from build123d import *

# Parameters (mm, degrees)
SKETCH2_W           = 25.4
SKETCH2_H           = 25.4
BOSS_EXTRUDE1_DEPTH = 25.4
SHELL1_T            = -4.7625
FILLET1_R           = 4.7625
SKETCH3_R           = 3.81
CUT_EXTRUDE1_DEPTH  = 25.4


with BuildPart() as part:
    # Sketch2 → Boss-Extrude1 (new body)
    with BuildSketch(Plane.XY):
        with Locations((12.7, 12.7)):
            Rectangle(SKETCH2_W, SKETCH2_H)
    extrude(amount=BOSS_EXTRUDE1_DEPTH)

    # Shell1
    shell1_openings = [part.faces().sort_by_distance(p)[0] for p in [
        (12.7, 12.7, 25.4),
        (12.7, 12.7, 0),
        (12.7, 25.4, 12.7),
        (25.4, 12.7, 12.7),
    ]]
    offset(amount=SHELL1_T, openings=shell1_openings, kind=Kind.INTERSECTION)

    # Fillet1
    fillet1_edges = [part.edges().sort_by_distance(p)[0] for p in [
        (25.4, 4.7625, 12.7),
        (4.7625, 25.4, 12.7),
    ]]
    fillet(fillet1_edges, radius=FILLET1_R - 0.0001)  # a hair under: the kernel refuses the full size

    # Sketch3 → Cut-Extrude1 (cut)
    with BuildSketch(Plane.ZY):
        with Locations((12.7, 12.7)):
            Circle(SKETCH3_R)
    cut_extrude1 = extrude(amount=-CUT_EXTRUDE1_DEPTH, mode=Mode.SUBTRACT)

    # Mirror1: Cut-Extrude1 across plane
    add(cut_extrude1.mirror(Plane(origin=(0, 0, 0), x_dir=(0, 0, 1), z_dir=(-0.7071067811865475, 0.7071067811865477, 0))), mode=Mode.SUBTRACT)


solid = part.part
Source: CAD feature listing. Evaluate the final solid. Frame: model axes, mm. A direction names the side the tool comes from. Coordinates: 2 decimals unless noted, no trailing zeros. Write each loop counter-clockwise with the first axis right and the second up, starting at its lowest first coordinate (ties: lowest second). Pieces come first, ordered by that corner, then holes. Notation, with made-up numbers: M 85.25,80.25 L 107.25,80.25 A18 ccw 107.25,90.25 Z; hole C 6,83.25 d4. An arc over 180 degrees is marked long. Use a Markdown table: item, result.
1) Reachability of faces 4 (the flat face through (4.762, 16, 15)), 5 (the flat face through (9.7, 0, 9.7)) from +Z, -Z, +X, -X, +Y, -Y: full face, straight path, thin tool, end or side. Return the list, or none.
Conclusion:
| item | result |
|---|---|
| face 4 | +Z, -Z, +X, +Y |
| face 5 | +Z, -Z, +X, -X, -Y |
2) Ray query, L1, parallel to Y at x = 11, z = 20.75; L2, parallel to Y at x = 3.35, z = 12.7; L3, parallel to Z at x = 12.25, y = 4. Return the intervals inside material, ascending.
Conclusion:
| item | result |
|---|---|
| L1 | y = 0 to 4.76 |
| L2 | y = 0 to 8.89, 16.51 to 24.02 |
| L3 | z = 0 to 8.92, 16.48 to 25.4 |
3) Section C-C, the plane z = 12.7. Give the number of separate pieces and of enclosed holes in the cut face, then the cut area to 3 significant figures.
Conclusion:
| item | result |
|---|---|
| separate pieces | 3 |
| enclosed holes | 0 |
| area | 137 mm^2 |
4) Mould query, pull axis Z, two halves, no side actions, for faces 1 (the cylindrical face through (24.04, 3.33, 12.52)), 2 (the flat face through (4, 7, 0)), 3 (the cylindrical face through (2.35, 10.38, 9.68)). Classes: pulls with the +Z half, pulls with the -Z half, needs draft (parallel to the pull), parting line crosses it, or undercut.
Conclusion:
| item | result |
|---|---|
| face 1 | needs draft |
| face 2 | pulls with the -Z half |
| face 3 | undercut |
5) First-contact query: pin 1 Ø4 at (y, z) = (22.5, 21.5) entering from +X; pin 2 Ø5 at (x, z) = (9.5, 11.5) entering from +Y; pin 3 Ø6 at (y, z) = (12.7, 12.7) entering from -X. Flat tips, straight axial feed; report the tip coordinate or a pass-through.
Conclusion:
| item | result |
|---|---|
| pin 1 | stops at x = 4.76 |
| pin 2 | stops at y = 4.76 |
| pin 3 | passes through |
6) Section A-A, the plane y = 12.7. Output: boundary loops of the cut face in (x, z).
Conclusion:
| item | result |
|---|---|
| outline | M 0,0 L 4.76,0 L 4.76,8.89 L 0,8.89 Z; M 0,16.51 L 4.76,16.51 L 4.76,25.4 L 0,25.4 Z |
